Model file for the job. Use its own axes, mm. Face numbers are marked on the shaded views. A direction names the side the tool comes from. Round coordinates to 2 decimals unless told otherwise and drop trailing zeros. Loops run counter-clockwise (first coordinate to the right, second up) from the corner with the lowest first, then second, coordinate; pieces in that order, holes last. Notation, with made-up numbers: (24, -7.5) -> (81, -7.5) arc R20 ccw to (81, 10.5) -> close; hole circle Ø8 at (-34, -9.75). An arc over 180 degrees is marked (long way). Use a Markdown table: item, result.
from build123d import *

# Parameters (mm, degrees)
SKETCH1_W                        = 228.6
SKETCH1_H                        = 165.1
SKETCH1_W_2                      = 203.2
SKETCH1_H_2                      = 139.7
FRAME_DEPTH                      = 19.05
SKETCH2_R                        = 2.159
FRONTWALL_MOUNTINGHOLES_DEPTH    = 7.112
SKETCH3_W                        = 12.7
SKETCH3_H                        = 10.16
BOSS_EXTRUDE2_DEPTH              = 8.89
SKETCH4_R                        = 1.5875
CUT_EXTRUDE2_DEPTH               = 148.609844184
SKETCH5_R                        = 1.5875
CUT_EXTRUDE3_DEPTH               = 12.7
FILLET3_R                        = 1.905
SKETCH6_R                        = 2.159
LINKAGE_RHS_MOUNTINGHOLES_DEPTH  = 7.112
SKETCH7_R                        = 2.159
LINKAGE_LHS_MOUNTINGHOLES_DEPTH  = 7.112
SKETCH11_W                       = 12.7
SKETCH11_H                       = 10.16
CUT_EXTRUDE6_DEPTH               = 0.381
FILLET2_R                        = 1.27
CHAMFER1_SIZE                    = 1.27
SKETCH12_R                       = 2.159
CASTER_WHEEL_MOUNT_DEPTH         = 7.112
SKETCH13_R                       = 2.159
FRONTBRACE_MOUNT_DEPTH           = 7.112
SKETCH14_R                       = 2.159
USB_HUB_SWITCH_MOUNT_HOLES_DEPTH = 7.112
FILLET4_R                        = 2.54


with BuildPart() as part:
    # Sketch1 → Frame (new body)
    with BuildSketch(Plane(origin=(0, 0, 0), x_dir=(1, 0, 0), z_dir=(0, 1, 0))):
        Rectangle(SKETCH1_W, SKETCH1_H)
        Rectangle(SKETCH1_W_2, SKETCH1_H_2, mode=Mode.SUBTRACT)
    extrude(amount=FRAME_DEPTH)

    # Sketch2 → FrontWall_mountingHoles (cut)
    with BuildSketch(Plane(origin=(0, 19.05, 0), x_dir=(1, 0, 0), z_dir=(0, 1, 0))):
        with Locations(Location((-95.25, 76.2, 0), (0, 0, 270))):
            Circle(SKETCH2_R)
        with Locations(Location((-107.95, 63.5, 0), (0, 0, 270))):
            Circle(SKETCH2_R)
        with Locations(Location((95.25, 76.2, 0), (0, 0, 90))):
            Circle(SKETCH2_R)
        with Locations(Location((107.95, 63.5, 0), (0, 0, 90))):
            Circle(SKETCH2_R)
    extrude(amount=-FRONTWALL_MOUNTINGHOLES_DEPTH, mode=Mode.SUBTRACT)

    # Sketch3 → Boss-Extrude2 (add)
    with BuildSketch(Plane.XY.offset(82.55)):
        with Locations((107.95, 13.97)):
            Rectangle(SKETCH3_W, SKETCH3_H)
        with Locations((0, 13.97)):
            Rectangle(SKETCH3_W, SKETCH3_H)
        with Locations((-107.95, 13.97)):
            Rectangle(SKETCH3_W, SKETCH3_H)
    extrude(amount=BOSS_EXTRUDE2_DEPTH)

    # Sketch4 → Cut-Extrude2 (cut, through all)
    with BuildSketch(Plane(origin=(0, 19.05, 0), x_dir=(1, 0, 0), z_dir=(0, 1, 0))):
        with Locations(Location((-107.95, -86.995, 0), (0, 0, 270))):
            Circle(SKETCH4_R)
        with Locations(Location((0, -86.995, 0), (0, 0, 270))):
            Circle(SKETCH4_R)
        with Locations(Location((107.95, -86.995, 0), (0, 0, 270))):
            Circle(SKETCH4_R)
    extrude(amount=-CUT_EXTRUDE2_DEPTH, mode=Mode.SUBTRACT)

    # Sketch5 → Cut-Extrude3 (cut)
    with BuildSketch(Plane.XY.offset(82.55)):
        with Locations((-20.32, 9.525)):
            Circle(SKETCH5_R)
        with Locations((-81.28, 9.525)):
            Circle(SKETCH5_R)
        with Locations(Location((81.28, 9.525, 0), (0, 0, 180))):
            Circle(SKETCH5_R)
        with Locations(Location((20.32, 9.525, 0), (0, 0, 180))):
            Circle(SKETCH5_R)
    extrude(amount=-CUT_EXTRUDE3_DEPTH, mode=Mode.SUBTRACT)

    # Fillet3
    fillet3_edges = [part.edges().sort_by_distance(p)[0] for p in [
        (101.6, 9.525, 69.85),
        (101.6, 9.525, -69.85),
        (-101.6, 9.525, -69.85),
        (-101.6, 9.525, 69.85),
    ]]
    fillet(fillet3_edges, radius=FILLET3_R)

    # Sketch6 → Linkage_RHS_MountingHoles (cut)
    with BuildSketch(Plane(origin=(0, 19.05, 0), x_dir=(1, 0, 0), z_dir=(0, 1, 0))):
        with Locations(Location((107.95, -4.445, 0), (0, 0, 270))):
            Circle(SKETCH6_R)
        with Locations(Location((107.95, -32.766, 0), (0, 0, 270))):
            Circle(SKETCH6_R)
        with Locations(Location((107.95, -42.164, 0), (0, 0, 270))):
            Circle(SKETCH6_R)
        with Locations(Location((107.95, -70.485, 0), (0, 0, 270))):
            Circle(SKETCH6_R)
    extrude(amount=-LINKAGE_RHS_MOUNTINGHOLES_DEPTH, mode=Mode.SUBTRACT)

    # Sketch7 → Linkage-LHS-MountingHoles (cut)
    with BuildSketch(Plane(origin=(0, 19.05, 0), x_dir=(1, 0, 0), z_dir=(0, 1, 0))):
        with Locations(Location((-107.95, 41.91, 0), (0, 0, 270))):
            Circle(SKETCH7_R)
        with Locations(Location((-107.95, 19.05, 0), (0, 0, 270))):
            Circle(SKETCH7_R)
        with Locations(Location((-107.95, -3.81, 0), (0, 0, 270))):
            Circle(SKETCH7_R)
    extrude(amount=-LINKAGE_LHS_MOUNTINGHOLES_DEPTH, mode=Mode.SUBTRACT)

    # Sketch11 → Cut-Extrude6 (cut)
    with BuildSketch(Plane.XY.offset(91.44)):
        with Locations((-107.95, 13.97)):
            Rectangle(SKETCH11_W, SKETCH11_H)
        with Locations((0, 13.97)):
            Rectangle(SKETCH11_W, SKETCH11_H)
        with Locations((107.95, 13.97)):
            Rectangle(SKETCH11_W, SKETCH11_H)
    extrude(amount=-CUT_EXTRUDE6_DEPTH, mode=Mode.SUBTRACT)

    # Fillet2
    fillet2_edges = [part.edges().sort_by_distance(p)[0] for p in [
        (101.6, 13.97, 82.55),
        (107.95, 8.89, 82.55),
        (-107.95, 8.89, 82.55),
        (-101.6, 13.97, 82.55),
        (6.35, 13.97, 82.55),
        (-6.35, 13.97, 82.55),
        (0, 8.89, 82.55),
    ]]
    fillet(fillet2_edges, radius=FILLET2_R)

    # Chamfer1
    chamfer1_edges = [part.edges().sort_by_distance(p)[0] for p in [
        (-114.3, 13.97, 91.059),
        (-101.6, 13.97, 91.059),
        (-107.95, 8.89, 91.059),
        (0, 8.89, 91.059),
        (-6.35, 13.97, 91.059),
        (6.35, 13.97, 91.059),
        (107.95, 8.89, 91.059),
        (101.6, 13.97, 91.059),
        (114.3, 13.97, 91.059),
    ]]
    chamfer(chamfer1_edges, length=CHAMFER1_SIZE)

    # Sketch12 → Caster_Wheel_Mount (cut)
    with BuildSketch(Plane(origin=(0, 19.05, 0), x_dir=(1, 0, 0), z_dir=(0, 1, 0))):
        with Locations(Location((-31.115, 76.2, 0), (0, 0, 270))):
            Circle(SKETCH12_R)
        with Locations(Location((31.115, 76.2, 0), (0, 0, 90))):
            Circle(SKETCH12_R)
        with Locations(Location((31.115, -76.2, 0), (0, 0, 270))):
            Circle(SKETCH12_R)
        with Locations(Location((-31.115, -76.2, 0), (0, 0, 90))):
            Circle(SKETCH12_R)
    extrude(amount=-CASTER_WHEEL_MOUNT_DEPTH, mode=Mode.SUBTRACT)

    # Sketch13 → FrontBrace_Mount (cut)
    with BuildSketch(Plane(origin=(0, 19.05, 0), x_dir=(1, 0, 0), z_dir=(0, 1, 0))):
        with Locations(Location((-12.7, 76.2, 0), (0, 0, 270))):
            Circle(SKETCH13_R)
        with Locations(Location((12.7, 76.2, 0), (0, 0, 90))):
            Circle(SKETCH13_R)
    extrude(amount=-FRONTBRACE_MOUNT_DEPTH, mode=Mode.SUBTRACT)

    # Sketch14 → USB_HUB_Switch_Mount_Holes (cut)
    with BuildSketch(Plane(origin=(0, 19.05, 0), x_dir=(1, 0, 0), z_dir=(0, 1, 0))):
        with Locations(Location((-107.95, -25.4, 0), (0, 0, 270))):
            Circle(SKETCH14_R)
        with Locations(Location((-107.95, -76.2, 0), (0, 0, 90))):
            Circle(SKETCH14_R)
    extrude(amount=-USB_HUB_SWITCH_MOUNT_HOLES_DEPTH, mode=Mode.SUBTRACT)

    # Fillet4
    fillet4_edges = [part.edges().sort_by_distance(p)[0] for p in [
        (-114.3, 3.81, 82.55),
        (114.3, 3.81, 82.55),
        (114.3, 8.518025612, 82.921974388),
        (-114.3, 8.518025612, 82.921974388),
        (114.3, 8.89, 86.8045),
        (-114.3, 8.89, 86.8045),
        (-114.3, 9.525, -82.55),
        (114.3, 9.525, -82.55),
    ]]
    fillet(fillet4_edges, radius=FILLET4_R)


solid = part.part
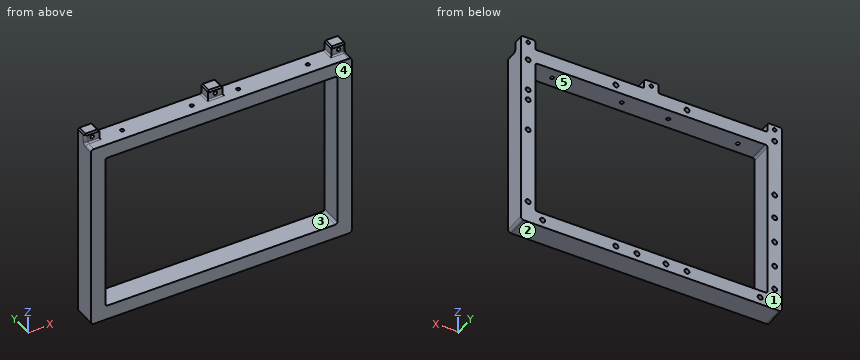
Q1. Flat gauge pins, fed straight in: pin 1 (9.5 mm diameter, centred on x = 22.5, y = 10.5, fed in from +Z); pin 2 (2.5 mm diameter, centred on x = -107.95, z = -41.91, fed in from +Y). Where does each tip first touch, or does it go through?
Results list:
| item | result |
|---|---|
| pin 1 | stops at z = 82.55 |
| pin 2 | stops at y = 11.94 |
Q2. Band-saw the part on C-C, the plane z = -3.5. Give the cut face in (x, y), plus the area to 3 significant figures.
Results list:
| item | result |
|---|---|
| outline | (-114.3, 0) -> (-101.6, 0) -> (-101.6, 19.05) -> (-114.3, 19.05) -> close; (101.6, 0) -> (114.3, 0) -> (114.3, 19.05) -> (101.6, 19.05) -> close |
| area | 484 mm² |
Q3. Band-saw the part on A-A, the plane x = 70.5. Give the cut face in (y, z), plus the area to 3 significant figures.
Results list:
| item | result |
|---|---|
| outline | (0, -82.55) -> (19.05, -82.55) -> (19.05, -69.85) -> (0, -69.85) -> close; (0, 69.85) -> (19.05, 69.85) -> (19.05, 82.55) -> (0, 82.55) -> close |
| area | 484 mm² |
Q4. Pull direction Z, two halves, no side cores. Call the marked faces 1, 2 and 3: released by +Z, released by -Z, zero draft, split by the parting line, or undercut.
Results list:
| item | result |
|---|---|
| face 1 | zero draft |
| face 2 | released by -Z |
| face 3 | undercut |
Q5. Tool access for the marked faces 4 and 5: list every direction of +Z, -Z, +X, -X, +Y, -Y with a clear straight run to the whole face (end or side of a thin tool).
Results list:
| item | result |
|---|---|
| face 4 | +Z, -Z, +X, -X, -Y |
| face 5 | +Y, -Y |
Q6. Band-saw the part on D-D, the plane y = 14.75. Give the number of separate pieces and of enclosed holes in the cut face, plus the area to 3 significant figures.
Results list:
| item | result |
|---|---|
| separate pieces | 1 |
| enclosed holes | 23 |
| area | 9,370 mm² |
Q7. Drill centre lines: L1, parallel to X at y = 13.5, z = 25.5; L2, parallel to Z at x = 54, y = 1.5; L3, parallel to X at y = 11.75, z = 21. Where is each one in solid material? Low to high. Write a range as from..to.
Results list:
| item | result |
|---|---|
| L1 | x = -114.3..-110.11, -105.79..-101.6, 101.6..114.3 |
| L2 | z = -82.55..-69.85, 69.85..82.55 |
| L3 | x = -114.3..-101.6, 101.6..114.3 |
Q8. Band-saw the part on B-B, the plane y = 3.5. Give the cut face in (x, z) (3 decimals).
Results list:
| item | result |
|---|---|
| outline | (-114.3, -80.01) arc R2.54 ccw to (-111.76, -82.55) -> (111.76, -82.55) arc R2.54 ccw to (114.3, -80.01) -> (114.3, 80.01) arc R2.54 ccw to (111.76, 82.55) -> (-111.76, 82.55) arc R2.54 ccw to (-114.3, 80.01) -> close; hole (-101.6, -67.945) arc R1.905 ccw to (-99.695, -69.85) -> (99.695, -69.85) arc R1.905 ccw to (101.6, -67.945) -> (101.6, 67.945) arc R1.905 ccw to (99.695, 69.85) -> (-99.695, 69.85) arc R1.905 ccw to (-101.6, 67.945) -> close |
